Could you check a few things on this model? Use its own coordinates, in mm. Face numbers are marked on the shaded views. A direction names the side the tool comes from. Give positions to 0.01 mm unless a question says otherwise; leave off trailing zeros. Loops run counter-clockwise (first coordinate to the right, second up) from the corner with the lowest first, then second, coordinate; pieces in that order, holes last. Notation, with made-up numbers: M -8.75,42 L 50.25,42 A21 cw 50.25,64 Z; hole C 5.5,-34.5 d2. An arc over 180 degrees is marked long. Use CSV: the item, a comma, the result in double quotes.
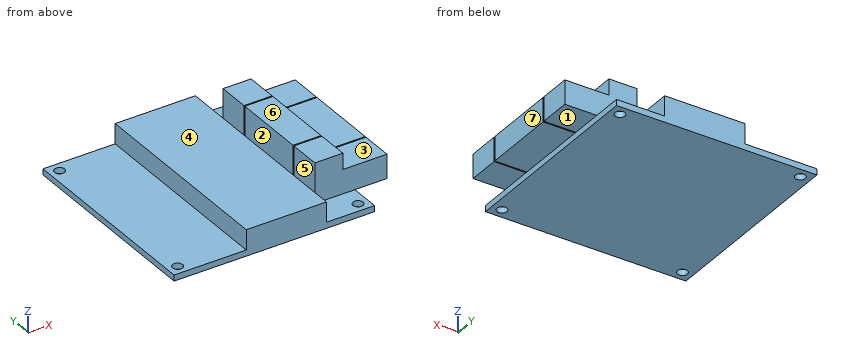
```python
from build123d import *

# Parameters (mm, degrees)
SKETCH_1_W          = 50
SKETCH_1_H          = 50
EXTRUDE_1_DEPTH     = 1.5
SKETCH_2_W          = 20
SKETCH_2_H          = 50
EXTRUDE_2_DEPTH     = 5
SKETCH_3_W          = 18
SKETCH_3_H          = 8
SKETCH_3_H_2        = 18.4
EXTRUDE_3_DEPTH     = 10
SKETCH_4_W          = 11
SKETCH_4_H          = 4
CUT_EXTRUDE_1_DEPTH = 56.022722579
SKETCH_5_R          = 1.25
CUT_EXTRUDE_2_DEPTH = 43.591078878


with BuildPart() as part:
    # 草图1 → 凸台-拉伸1 (new body)
    with BuildSketch(Plane.XY):
        Rectangle(SKETCH_1_W, SKETCH_1_H)
    extrude(amount=EXTRUDE_1_DEPTH)

    # 草图2 → 凸台-拉伸2 (add)
    with BuildSketch(Plane.XY.offset(1.5)):
        with Locations((3, 0)):
            Rectangle(SKETCH_2_W, SKETCH_2_H)
    extrude(amount=EXTRUDE_2_DEPTH)

    # 草图3 → 凸台-拉伸3 (add)
    with BuildSketch(Plane.XY.offset(1.5)):
        with Locations((24, 13.5)):
            Rectangle(SKETCH_3_W, SKETCH_3_H)
        with Locations((24, 0)):
            Rectangle(SKETCH_3_W, SKETCH_3_H_2)
        with Locations((24, -13.5)):
            Rectangle(SKETCH_3_W, SKETCH_3_H)
    extrude(amount=EXTRUDE_3_DEPTH)

    # 草图4 → 切除-拉伸1 (cut, through all)
    with BuildSketch(Plane.XZ.offset(17.5)):
        with Locations((27.5, 9.5)):
            Rectangle(SKETCH_4_W, SKETCH_4_H)
    extrude(amount=-CUT_EXTRUDE_1_DEPTH, mode=Mode.SUBTRACT)

    # 草图5 → 切除-拉伸2 (cut, through all)
    with BuildSketch(Plane.XY.offset(1.5)):
        with Locations((-22.5, 22.5)):
            Circle(SKETCH_5_R)
        with Locations((22.5, 22.5)):
            Circle(SKETCH_5_R)
        with Locations((22.5, -22.5)):
            Circle(SKETCH_5_R)
        with Locations((-22.5, -22.5)):
            Circle(SKETCH_5_R)
    extrude(amount=-CUT_EXTRUDE_2_DEPTH, mode=Mode.SUBTRACT)


solid = part.part
```
1. I want a section at D-D, the plane y = -4.5. List the corners of the cut face in (x, z) for me.
Outcome:
outline,"M -25,0 L 25,0 L 25,1.5 L 33,1.5 L 33,7.5 L 22,7.5 L 22,11.5 L 15,11.5 L 15,1.5 L 13,1.5 L 13,6.5 L -7,6.5 L -7,1.5 L -25,1.5 Z"
2. I want a section at A-A, the plane x = -22.5. List the corners of the cut face in (y, z) for me, then the cut area to 3 significant figures.
Outcome:
outline,"M -25,0 L -23.75,0 L -23.75,1.5 L -25,1.5 Z; M -21.25,0 L 21.25,0 L 21.25,1.5 L -21.25,1.5 Z; M 23.75,0 L 25,0 L 25,1.5 L 23.75,1.5 Z"
area,"67.5 mm2"
3. If we mould it in two halves opening along X, with no side actions, what happens to the marked faces 5, 6 and 7? For each: +X half, -X half, draft (parallel to the pull), parting line (faces both ways), or undercut.
Outcome:
face 5,"undercut"
face 6,"draft"
face 7,"+X half"
4. I want a section at C-C, the plane y = 22.5. List the corners of the cut face in (x, z) for me.
Outcome:
outline,"M -25,0 L -23.75,0 L -23.75,1.5 L -25,1.5 Z; M -21.25,0 L 21.25,0 L 21.25,1.5 L 13,1.5 L 13,6.5 L -7,6.5 L -7,1.5 L -21.25,1.5 Z; M 23.75,0 L 25,0 L 25,1.5 L 23.75,1.5 Z"
5. Which directions (+Z, -Z, +X, -X, +Y, -Y) give clear straight access to the entire face, cutting with the end or side of a thin tool? Please do the marked faces 1, 2, 3 and 4.
Outcome:
face 1,"-Z, +X, +Y, -Y"
face 2,"+Z, +Y, -Y"
face 3,"+Z, +X, +Y, -Y"
face 4,"+Z, -X, +Y, -Y"
6. Please list where these lines run through material, in increasing order: line 1 (Y direction, x = 22.5, z = 1); line 2 (X direction, y = -5, z = 4); line 3 (Z direction, x = -21.5, y = 2).
Outcome:
line 1,"-25 to -23.75, -21.25 to 21.25, 23.75 to 25"
line 2,"-7 to 13, 15 to 33"
line 3,"0 to 1.5"
7. I want a section at B-B, the plane z = 3. List the corners of the cut face in (x, y) for me, then the cut area to 3 significant figures.
Outcome:
outline,"M -7,-25 L 13,-25 L 13,25 L -7,25 Z; M 15,-17.5 L 33,-17.5 L 33,-9.5 L 15,-9.5 Z; M 15,-9.2 L 33,-9.2 L 33,9.2 L 15,9.2 Z; M 15,9.5 L 33,9.5 L 33,17.5 L 15,17.5 Z"
area,"1,620 mm2"
8. I'm going to push flat-ended pins straight in: pin 1 Ø5 at (x, y) = (-0.5, -6.5) entering from +Z; pin 2 Ø4 at (y, z) = (12, 5) entering from -X; pin 3 Ø5 at (x, z) = (-10, 5.5) entering from -Y; pin 4 Ø1.2 at (y, z) = (-13, 9) entering from +X. Where does each tip first touch, or does it pass through?
Outcome:
pin 1,"z = 6.5"
pin 2,"x = -7"
pin 3,"through"
pin 4,"x = 22"
